Work out the finished part from the listing and answer in its coordinate system (mm). A direction names the side the tool comes from. Coordinates: 2 decimals unless noted, no trailing zeros. Order: outer loops, then holes, each group sorted by start corner. A loop starts at its lowest first (then second) coordinate and runs counter-clockwise, first axis right, second up. Notation, with made-up numbers: (38, 25.25) - (59, 25.25) arc R21 cw to (59, 42.25) - close; hole circle Ø11 at (72.5, 14.25). An arc over 180 degrees is marked (long way). Answer as a JSON object with one key per item and string values. Group by question number.
1) A tool of negligible diameter and unlimited length cuts with its end or side. For faces 4 (the face through (-103, 219, 0)), 5 (the face through (-102.5, 218, -7)), 6 (the face through (-112.5, 223, -1)), 7 (the face through (-112, 218, -12)), from which of +Z, -Z, +X, -X, +Y, -Y can it reach the whole face along a straight path? Write none if from no direction.
2) Section C-C (y = 217) is taken. Give the vertices of the cut face in (x, z), plus the area to 3 significant figures.
3) The mould has two halves that part along Y. Classify faces 1 (the face through (-111, 226.5, 0)), 2 (the face through (-113, 218, 11)), 3 (the face through (-114, 225.5, -1)): released by +Y, released by -Y, zero draft, split by the parting line, or undercut.
4) Section B-B (z = -0.5) is taken. Give the vertices of the cut face in (x, y).
5) Section A-A (y = 224.75) is taken. Give the vertices of the cut face in (x, z).
6) Section D-D (x = -118) is taken. Give the vertices of the cut face in (y, z), plus the area to 3 significant figures.
7) Each of these flat-tipped pins is pushed along its axis until it touches: P1, Ø5, axis at y = 224, z = 1, coming from the -X side; P2, Ø0.5, axis at x = -102.5, z = 0.5, coming from the +Y side. Where does it stop, or does it pass through?
8) Find the intervals of material crossed by line 1 along Z through (x, y) = (-99.5, 222.25); line 2 along Y through (x, z) = (-114, -2.25); line 3 along X through (y, z) = (214, -5), in increasing order.
Autodesk Inventor part; units mm, degrees
ref_plane "YZ Plane" through (0, 0, 0) normal (1, 0, 0) x (0, 1, 0)
ref_plane "XZ Plane" through (0, 0, 0) normal (0, 1, 0) x (-1, 0, 0)
ref_plane "XY Plane" through (0, 0, 0) normal (0, 0, 1) x (1, 0, 0)
sketch "Sketch1" plane through (0, 0, 0) normal (0, 1, 0) x (-1, 0, 0)
  line L0 (162, 9) -> (164.5, 9)
  line L1 (164.5, -10) -> (162, -10)
  line L2 (162, -10) -> (162, 9)
  line L3 (190, 11) -> (161, 11)
  line L4 (160, 10) -> (160, -11)
  line L5 (161, -12) -> (190, -12)
  line L6 (164.5, 7) -> (165.5, 7)
  line L7 (164.5, -8) -> (165.5, -8)
  line L8 (165.5, 7) -> (165.5, 5.5)
  line L9 (165.5, 5.5) -> (165, 5.5)
  line L10 (165.5, -8) -> (165.5, -6.5)
  line L11 (165.5, -6.5) -> (165, -6.5)
  line L12 (164.5, 7) -> (164.5, 9)
  line L13 (165, 5.5) -> (165, -6.5)
  line L14 (164.5, -8) -> (164.5, -10)
  arc A0 (161, 11) -> (160, 10) centre (161, 10) ccw
  arc A1 (160, -11) -> (161, -12) centre (161, -11) ccw
  line L15 (190, 11) -> (190, -12)
  point P0 (0, 0)
  dimension "d0" = 19
  dimension "d1" = 2.5
  dimension "d3" = 2
  dimension "d4" = 2
  dimension "d5" = 2
  dimension "d7" = 1
  dimension "d8" = 15
  dimension "d10" = 1.5
  dimension "d11" = 1.5
  dimension "d12" = 1
  dimension "d22" = 4
  dimension "d28" = 3
  dimension "d36" = 30
  dimension "d46" = 11
  dimension "d48" = 190
extrude "Extrusion1" add sketch "Sketch1" along normal blind 16.5
sketch "Sketch5" plane through (0, 16.5, 0) normal (0, 1, 0) x (1, 0, 0)
  line L0 (-165, -3.25) -> (-166, -3.25)
  line L1 (-166, -3.25) -> (-166, 3.25)
  line L2 (-166, 3.25) -> (-165, 3.25)
  line L3 (-165, 3.25) -> (-165, -3.25)
  line L4 (-165, -5.5) -> (-165, 6.5)
  line L5 (-190, -11) -> (-161, -11)
  point P0 (0, 0)
  point P1 (-21.5, -2)
  dimension "d15" = 1
  dimension "d16" = 6.5
  dimension "d17" = 0
  dimension "d18" = 7.75
extrude "Extrusion2" cut sketch "Sketch5" against normal blind 15
move or copy body "Move Body2" bodies to move or copy 1 copy no translate (63, 210, 0)
fillet "Fillet1" [suppressed]
sketch "Sketch21" plane through (-127, 226.5, 11) normal (0, 1, 0) x (1, 0, 0)
  circle A0 centre (0, 11.5) radius 11
  line L0 (24, 7.75) -> (24, 14.25)
  line L1 (29, 23) -> (0, 23)
  circle A1 centre (0, 11.5) radius 13
  line L2 (0, 0) -> (29, 0)
  point P0 (127, 11)
  point P1 (6.0622, 0)
  dimension "d61" = 26
  dimension "d56" = 22
  dimension "d57" = 24
  dimension "d58" = 11.5
extrude "Extrusion4" cut sketch "Sketch21" against normal up to next contours A0
sketch "Sketch24" plane through (-98, 210, -12) normal (0, 0, -1) x (-1, 0, 0)
  line L0 (17, 1) -> (14.5, 1)
  line L1 (14.5, 1) -> (14.5, 5.5)
  line L2 (14.5, 5.5) -> (17, 5.5)
  line L3 (17, 5.5) -> (17, 1)
  line L4 (17, 11.1) -> (14.5, 11.1)
  line L5 (14.5, 11.1) -> (14.5, 15.5)
  line L6 (14.5, 15.5) -> (17, 15.5)
  line L7 (17, 15.5) -> (17, 11.1)
  line L8 (29, 0) -> (0, 0)
  line L9 (29, 0) -> (29, 16.5)
  line L10 (0, 16.5) -> (29, 16.5)
  point P0 (-98, -210)
  dimension "d68" = 2.5
  dimension "d69" = 4.5
  dimension "d70" = 2.5
  dimension "d71" = 4.4
  dimension "d72" = 1
  dimension "d73" = 12
  dimension "d74" = 12
  dimension "d75" = 1
extrude "Extrusion5" cut sketch "Sketch24" against normal up to next
fillet "Fillet2" radius 1 10 edges at (-97.2929, 210, -11.7071) (-97, 210, -0.5) (-97.2929, 210, 10.7071) (-112.5, 210, 11) (-112.5, 210, -12) (-97.2929, 226.5, -11.7071) (-97, 226.5, -0.5) (-97.2929, 226.5, 10.7071) (-112.5, 226.5, 11) (-112.5, 226.5, -12)
properties part number "rear_light_mount"
Report:
{
 "1": {"face 4": "+Y", "face 5": "+Y, -Y", "face 6": "+Z, -Z", "face 7": "-Z, +X, -X, +Y, -Y"},
 "2": {"outline": "(-127, -12) - (-98, -12) arc R1 ccw to (-97, -11) - (-97, 10) arc R1 ccw to (-98, 11) - (-127, 11) - (-127, 10.5) arc R11 cw to (-127, -11.5) - close; hole (-103, -3.25) - (-102, -3.25) - (-102, -6.5) - (-102.5, -6.5) - (-102.5, -8) - (-101.5, -8) - (-101.5, -10) - (-99, -10) - (-99, 9) - (-101.5, 9) - (-101.5, 7) - (-102.5, 7) - (-102.5, 5.5) - (-102, 5.5) - (-102, 3.25) - (-103, 3.25) - close", "area": "437 mm²"},
 "3": {"face 1": "released by +Y", "face 2": "zero draft", "face 3": "undercut"},
 "4": {"outline": "(-116, 210) - (-102, 210) - (-102, 211.5) - (-103, 211.5) - (-103, 226.5) - (-116, 226.5) - close; (-99, 210) - (-98, 210) arc R1 ccw to (-97, 211) - (-97, 225.5) arc R1 ccw to (-98, 226.5) - (-99, 226.5) - close; hole (-115, 211) - (-112.5, 211) - (-112.5, 215.5) - (-115, 215.5) - close; hole (-115, 221.1) - (-112.5, 221.1) - (-112.5, 225.5) - (-115, 225.5) - close"},
 "5": {"outline": "(-127, -12) - (-115, -12) - (-115, 11) - (-127, 11) - (-127, 10.5) arc R11 cw to (-127, -11.5) - close; (-112.5, -12) - (-98, -12) arc R1 ccw to (-97, -11) - (-97, 10) arc R1 ccw to (-98, 11) - (-112.5, 11) - close; hole (-103, -3.25) - (-102, -3.25) - (-102, -6.5) - (-102.5, -6.5) - (-102.5, -8) - (-101.5, -8) - (-101.5, -10) - (-99, -10) - (-99, 9) - (-101.5, 9) - (-101.5, 7) - (-102.5, 7) - (-102.5, 5.5) - (-102, 5.5) - (-102, 3.25) - (-103, 3.25) - close"},
 "6": {"outline": "(210, -11) arc R1 ccw to (211, -12) - (225.5, -12) arc R1 ccw to (226.5, -11) - (226.5, -6.82) - (210, -6.82) - close; (210, 5.82) - (226.5, 5.82) - (226.5, 10) arc R1 ccw to (225.5, 11) - (211, 11) arc R1 ccw to (210, 10) - close", "area": "170 mm²"},
 "7": {"P1": "stops at x = -116.75", "P2": "stops at y = 211.5"},
 "8": {"line 1": "z = -12 to -10, 9 to 11", "line 2": "y = 210 to 211, 215.5 to 221.1, 225.5 to 226.5", "line 3": "x = -116.96 to -115, -112.5 to -102, -99 to -97"}
}
